Can you work these out from the model? Positions are in its coordinate system, mm. A direction names the side the tool comes from. Round coordinates to 2 decimals unless told otherwise and drop trailing zeros. Order: outer loops, then holes, each group sorted by start corner. A loop starts at its lowest first (then second) coordinate and runs counter-clockwise, first axis right, second up.
from build123d import *


with BuildPart() as part:
    # 草圖1 → 旋轉1 (revolve)
    with BuildSketch(Plane.XY):
        with BuildLine():
            Line((0, 5), (0, 12))
            Line((0, 12), (1, 13))
            Line((1, 13), (8, 13))
            Line((8, 13), (10, 10))
            Line((10, 10), (45, 20))
            Line((45, 20), (55, 20))
            Line((55, 20), (55, 15))
            Line((55, 15), (23.556757793, 7.853808589))
            ThreePointArc((23.556757793, 7.853808589), (22.436912604, 7.151243881), (22, 5.903542878))
            Line((22, 5.903542878), (22, 5))
            Line((22, 5), (0, 5))
        make_face()
    revolve(axis=Axis((0, 0, 0), (1, 0, 0)))


solid = part.part
(1) I want a section at A-A, the plane z = 0. List the corners of the cut face in (x, y) for me, plus the area to 3 significant figures.
(2) I want a section at D-D, the plane x = 19.5. List the corners of the cut face in (y, z) for me, plus the area to 3 significant figures.
(3) I'm going to push flat-ended pins straight in: pin 1 Ø8 at (x, z) = (39, 13.5) entering from +Y; pin 2 Ø5 at (x, y) = (17.5, -9) entering from +Z; pin 3 Ø2 at (x, z) = (36, -7) entering from -Y; pin 4 Ø6 at (y, z) = (-0.5, 0) entering from +X. Where does each tip first touch, or does it pass through?
(4) I want a section at C-C, the plane x = 27. List the corners of the cut face in (y, z) for me.
(5) If we mould it in two halves opening along X, with no side actions, what happens to faces 5 (the face through (0, -5.2, 0.2)), 6 (the face through (9.903, -8.051, -6.173)), 7 (the face through (50.07, -4.336, -19.524)), 8 (the face through (55, 3, 15))? For each: pulls with the +X half, pulls with the -X half, needs draft (parallel to the pull), parting line crosses it, or undercut.
(6) On a 3-axis mill with a long thin cutter (end or side, diameter ignored), from which of +Z, -Z, +X, -X, +Y, -Y can I reach the whole of each face in a straight line? I mean faces 1 (the face through (10.85, -1.08, -4.88)), 2 (the face through (23.856, 13.314, 4.193)), 3 (the face through (4.549, -10.316, -7.91)), 4 (the face through (22, -4.4, 2.7)). Say none if no direction works.
(7) Please list where these lines run through material, in increasing order: probe 1 along Z at (x, y) = (4.75, 0); probe 2 along Z at (x, y) = (21, -2); probe 3 along Y at (x, z) = (52, -11.5).
Ans:
1. outline: (0, -12) - (1, -13) - (8, -13) - (10, -10) - (45, -20) - (55, -20) - (55, -15) - (23.56, -7.85) arc R2 cw to (22, -5.9) - (22, -5) - (0, -5) - close; (0, 5) - (22, 5) - (22, 5.9) arc R2 cw to (23.56, 7.85) - (55, 15) - (55, 20) - (45, 20) - (10, 10) - (8, 13) - (1, 13) - (0, 12) - close
1. area: 741 mm2
2. outline: circle Ø25.43 at (0, 0); hole circle Ø10 at (0, 0)
2. area: 429 mm2
3. pin 1: stops at y = 15.97
3. pin 2: stops at z = 10.47
3. pin 3: stops at y = -16.47
3. pin 4: passes through
4. outline: circle Ø29.71 at (0, 0); hole circle Ø17.27 at (0, 0)
5. face 5: pulls with the -X half
5. face 6: undercut
5. face 7: needs draft
5. face 8: pulls with the +X half
6. face 1: +X, -X
6. face 2: none
6. face 3: -X
6. face 4: +X
7. probe 1: z = -13 to -5, 5 to 13
7. probe 2: z = -12.99 to -4.58, 4.58 to 12.99
7. probe 3: y = -16.36 to -8.53, 8.53 to 16.36
